Model file for the job. Use its own axes, mm. Face numbers are marked on the shaded views. A direction names the side the tool comes from. Round coordinates to 2 decimals unless told otherwise and drop trailing zeros. Loops run counter-clockwise (first coordinate to the right, second up) from the corner with the lowest first, then second, coordinate; pieces in that order, holes last. Notation, with made-up numbers: M -4,14.5 L 20,14.5 A33 ccw 20,42.5 Z; hole C -17,29.25 d11. An arc over 180 degrees is marked long. Answer in a Markdown table with one row per item.
from build123d import *

# Parameters (mm, degrees)
CYLINDER033_R     = 1
CYLINDER033_DEPTH = 20
CYLINDER032_R     = 1
CYLINDER032_DEPTH = 20
CYLINDER012_R     = 5
CYLINDER012_DEPTH = 10
BOX003_W          = 8
BOX003_H          = 27
BOX003_DEPTH      = 20
BOX002_W          = 5.5
BOX002_H          = 5.5
BOX002_DEPTH      = 3
CYLINDER002_R     = 1.6
CYLINDER002_DEPTH = 5
CYLINDER003_R     = 2.75
CYLINDER003_DEPTH = 3
BOX001_W          = 5.5
BOX001_H          = 5.5
BOX001_DEPTH      = 3
CYLINDER_R        = 1.6
CYLINDER_DEPTH    = 5
CYLINDER001_R     = 2.75
CYLINDER001_DEPTH = 3
BOX_W             = 8
BOX_H             = 42
BOX_DEPTH         = 5


with BuildPart() as cylinder033:
    # Cylinder033 → Cylinder033 (new body)
    with BuildSketch(Plane(origin=(-15, 5.75, 9.75), x_dir=(0, 0, -1), z_dir=(1, 0, 0))):
        Circle(CYLINDER033_R)
    extrude(amount=CYLINDER033_DEPTH)


with BuildPart() as fusion020:
    # Cylinder032 → Cylinder032 (new body)
    with BuildSketch(Plane(origin=(-15, -5.75, 9.75), x_dir=(0, 0, -1), z_dir=(1, 0, 0))):
        Circle(CYLINDER032_R)
    extrude(amount=CYLINDER032_DEPTH)

    # Fusion020: union Cylinder033
    add(cylinder033.part)


with BuildPart() as cylinder012:
    # Cylinder012 → Cylinder012 (new body)
    with BuildSketch(Plane(origin=(-12.5, 7.5, 19.5), x_dir=(0, 0, -1), z_dir=(1, 0, 0))):
        Circle(CYLINDER012_R)
    extrude(amount=CYLINDER012_DEPTH)


with BuildPart() as cube003:
    # Box003 → Box003 (new body)
    with BuildSketch(Plane(origin=(-11.5, -13.5, 5), x_dir=(1, 0, 0), z_dir=(0, 0, 1))):
        with Locations((4, 13.5)):
            Rectangle(BOX003_W, BOX003_H)
    extrude(amount=BOX003_DEPTH)


with BuildPart() as cube002:
    # Box002 → Box002 (new body)
    with BuildSketch(Plane(origin=(-10.25, -24, 7), x_dir=(1, 0, 0), z_dir=(0, 0, 1))):
        with Locations((2.75, 2.75)):
            Rectangle(BOX002_W, BOX002_H)
    extrude(amount=BOX002_DEPTH)


with BuildPart() as cylinder002:
    # Cylinder002 → Cylinder002 (new body)
    with BuildSketch(Plane.XY):
        Circle(CYLINDER002_R)
    extrude(amount=CYLINDER002_DEPTH)


with BuildPart() as fusion003:
    # Cylinder003 → Cylinder003 (new body)
    with BuildSketch(Plane.XY.offset(2)):
        Circle(CYLINDER003_R)
    extrude(amount=CYLINDER003_DEPTH)

    # Fusion001: union Cylinder002
    add(cylinder002.part)


with BuildPart() as fusion003_1:
    # Fusion001 placement: moved
    add(fusion003.part.moved(Location((-7.5, -18.5, 5))))

    # Fusion003: union Cube002
    add(cube002.part)


with BuildPart() as cube001:
    # Box001 → Box001 (new body)
    with BuildSketch(Plane(origin=(-10.25, 18.5, 7), x_dir=(1, 0, 0), z_dir=(0, 0, 1))):
        with Locations((2.75, 2.75)):
            Rectangle(BOX001_W, BOX001_H)
    extrude(amount=BOX001_DEPTH)


with BuildPart() as cylinder:
    # Cylinder → Cylinder (new body)
    with BuildSketch(Plane.XY):
        Circle(CYLINDER_R)
    extrude(amount=CYLINDER_DEPTH)


with BuildPart() as fusion004:
    # Cylinder001 → Cylinder001 (new body)
    with BuildSketch(Plane.XY.offset(2)):
        Circle(CYLINDER001_R)
    extrude(amount=CYLINDER001_DEPTH)

    # Fusion: union Cylinder
    add(cylinder.part)


with BuildPart() as fusion004_1:
    # Fusion placement: moved
    add(fusion004.part.moved(Location((-7.6, 18.5, 5))))

    # Fusion002: union Cube001
    add(cube001.part)

    # Fusion004: union Fusion003
    add(fusion003_1.part)


with BuildPart() as holder:
    # Box → Box (new body)
    with BuildSketch(Plane(origin=(-11.5, -21, 5), x_dir=(1, 0, 0), z_dir=(0, 0, 1))):
        with Locations((4, 21)):
            Rectangle(BOX_W, BOX_H)
    extrude(amount=BOX_DEPTH)

    # Cut: cut Fusion004
    add(fusion004_1.part, mode=Mode.SUBTRACT)

    # Fusion005: union Cube003
    add(cube003.part)

    # Cut002: cut Cylinder012
    add(cylinder012.part, mode=Mode.SUBTRACT)

    # Cut009: cut Fusion020
    add(fusion020.part, mode=Mode.SUBTRACT)


with BuildPart() as holder_1:
    # Cut009 placement: moved
    add(holder.part.moved(Location((0, 0, 1))))


solid = holder_1.part
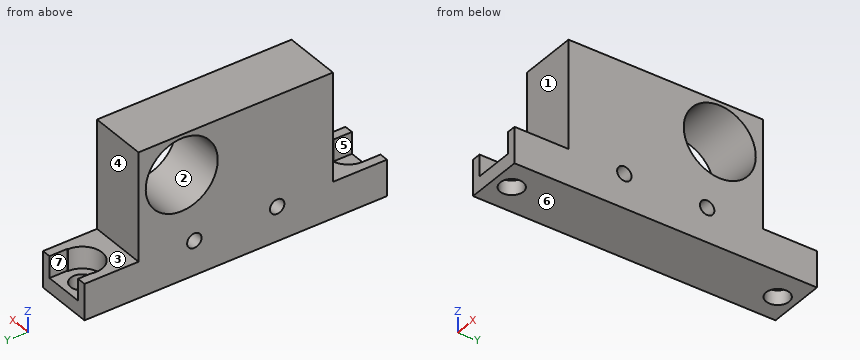
1. Saw through at D-D (x = -7.5). Write the cut outline in (y, z).
Verdict:
| item | result |
|---|---|
| outline | M -21,6 L -20.1,6 L -20.1,8 L -21,8 Z; M -16.9,6 L 16.9,6 L 16.9,8 L 15.75,8 L 15.75,11 L 13.5,11 L 13.5,26 L -13.5,26 L -13.5,11 L -15.75,11 L -15.75,8 L -16.9,8 Z; M 20.1,6 L 21,6 L 21,8 L 20.1,8 Z; hole C -5.75,10.75 d2; hole C 7.5,20.5 d10; hole C 5.75,10.75 d2 |
2. Wall check: probe 1 along Y at (x, z) = (-7.6, 7.1); probe 2 along Z at (x, y) = (-10, 7.5); probe 3 along Y at (x, z) = (-5.75, 20.5). Give the ranges that are in metal, low to high.
Verdict:
| item | result |
|---|---|
| probe 1 | y = -21 to -20.1, -16.9 to 16.9, 20.1 to 21 |
| probe 2 | z = 6 to 15.5, 25.5 to 26 |
| probe 3 | y = -13.5 to 2.5, 12.5 to 13.5 |
3. Saw through at C-C (y = -5.75). Write the cut outline in (x, z), and give its area (3 significant figures).
Verdict:
| item | result |
|---|---|
| outline | M -11.5,6 L -3.5,6 L -3.5,9.75 L -11.5,9.75 Z; M -11.5,11.75 L -3.5,11.75 L -3.5,26 L -11.5,26 Z |
| area | 144 mm² |
4. Pin check, flat tips, straight feed: pin 1 (2 mm diameter, centred on x = -9, y = -18, fed in from +Z); pin 2 (4 mm diameter, centred on x = -9, y = 17.5, fed in from +Z); pin 3 (4 mm diameter, centred on x = -5.5, z = 17.5, fed in from -Y). Stop position of each tip, or through.
Verdict:
| item | result |
|---|---|
| pin 1 | stops at z = 8 |
| pin 2 | stops at z = 11 |
| pin 3 | stops at y = -13.5 |
5. Tool access for the marked faces 5, 6 and 7: list every direction of +Z, -Z, +X, -X, +Y, -Y with a clear straight run to the whole face (end or side of a thin tool).
Verdict:
| item | result |
|---|---|
| face 5 | +Z, -Y |
| face 6 | -Z, +X, -X, +Y, -Y |
| face 7 | +Z, +Y |
6. Mould opens along Y. For the marked faces 1, 2, 3 and 4 say: +Y half, -Y half, draft (parallel to the pull), parting line (faces both ways), or undercut.
Verdict:
| item | result |
|---|---|
| face 1 | -Y half |
| face 2 | undercut |
| face 3 | draft |
| face 4 | +Y half |
7. Saw through at A-A (z = 23.5). Write the cut outline in (x, y), and give its area (3 significant figures).
Verdict:
| item | result |
|---|---|
| outline | M -11.5,-13.5 L -3.5,-13.5 L -3.5,3.5 L -11.5,3.5 Z; M -11.5,11.5 L -3.5,11.5 L -3.5,13.5 L -11.5,13.5 Z |
| area | 152 mm² |
8. Saw through at B-B (x = -4.25). Write the cut outline in (y, z), and give its area (3 significant figures).
Verdict:
| item | result |
|---|---|
| outline | M -21,6 L 21,6 L 21,11 L 13.5,11 L 13.5,26 L -13.5,26 L -13.5,11 L -21,11 Z; hole C -5.75,10.75 d2; hole C 7.5,20.5 d10; hole C 5.75,10.75 d2 |
| area | 530 mm² |
